from build123d import *

# Parameters (mm, degrees)
BOSS_EXTRUDE1_DEPTH = 40
FILLET1_R           = 20
SKETCH4_R           = 7.5
CUT_EXTRUDE1_DEPTH  = 40
CHAMFER1_SIZE       = 1


with BuildPart() as part:
    # Sketch3 → Boss-Extrude1 (new body)
    with BuildSketch(Plane.XY):
        with BuildLine():
            Line((-38.729833462, -5), (-100, -5))
            Line((-100, -5), (-100, 5))
            Line((-100, 5), (-38.729833462, 5))
            ThreePointArc((-38.729833462, 5), (-32.606109105, 7.09430585), (-29.047375097, 12.5))
            ThreePointArc((-29.047375097, 12.5), (0, 35), (29.047375097, 12.5))
            ThreePointArc((29.047375097, 12.5), (32.606109105, 7.09430585), (38.729833462, 5))
            Line((38.729833462, 5), (100, 5))
            Line((100, 5), (100, -5))
            Line((100, -5), (38.729833462, -5))
            ThreePointArc((38.729833462, -5), (32.606109105, -2.90569415), (29.047375097, 2.5))
            ThreePointArc((29.047375097, 2.5), (0, 25), (-29.047375097, 2.5))
            ThreePointArc((-29.047375097, 2.5), (-32.606109105, -2.90569415), (-38.729833462, -5))
        make_face()
    extrude(amount=BOSS_EXTRUDE1_DEPTH)

    # Fillet1
    fillet1_edges = [part.edges().sort_by_distance(p)[0] for p in [
        (100, 0, 0),
        (100, 0, 40),
        (-100, 0, 0),
        (-100, 0, 40),
    ]]
    fillet(fillet1_edges, radius=FILLET1_R - 0.0001)  # a hair under: the kernel refuses the full size

    # Sketch4 → Cut-Extrude1 (cut)
    with BuildSketch(Plane(origin=(0, 5, 0), x_dir=(1, 0, 0), z_dir=(0, 1, 0))):
        with Locations(Location((80, -20, 0), (0, 0, 180))):
            Circle(SKETCH4_R)
        with Locations(Location((-80, -20, 0), (0, 0, 180))):
            Circle(SKETCH4_R)
    extrude(amount=-CUT_EXTRUDE1_DEPTH, mode=Mode.SUBTRACT)

    # Chamfer1
    chamfer1_edges = [part.edges().sort_by_distance(p)[0] for p in [
        (87.5, 5, 20),
        (-72.5, 5, 20),
    ]]
    chamfer(chamfer1_edges, length=CHAMFER1_SIZE)


solid = part.part
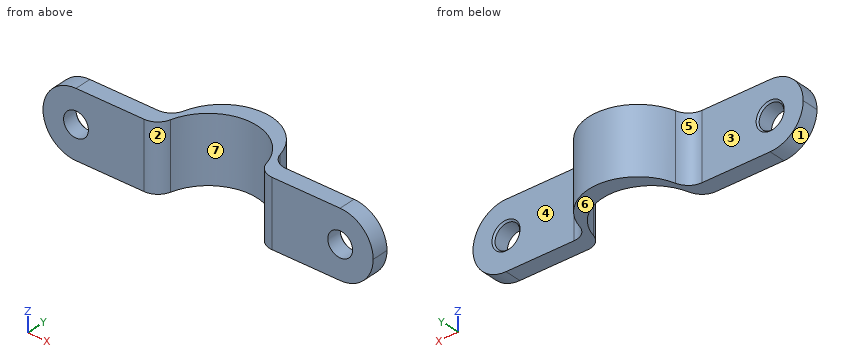
For this review, take the finished solid that the model builds, in its own axes (mm). Face numbers are marked on the shaded views. A direction names the side the tool comes from. Give positions to 0.01 mm unless a question says otherwise; leave off trailing zeros. Write each loop counter-clockwise with the first axis right and the second up, starting at its lowest first coordinate (ties: lowest second). Pieces come first, ordered by that corner, then holes. Notation, with made-up numbers: (-33, -12.75) -> (-12, -12.75) arc R15 cw to (-12, 5.25) -> close; hole circle Ø10 at (52, 71). An arc over 180 degrees is marked (long way). Use CSV: the item, a comma, the result in double quotes.
Q1. Take a section at B-B, the plane y = -1.5. State how many separate pieces and enclosed holes the cut face has, then the cut area to 3 significant figures.
Conclusion:
separate pieces,"2"
enclosed holes,"2"
area,"4,810 mm2"
Q2. Mouldability with a two-part tool opening along X and no side actions: class the marked faces 5, 6 and 7 as pulls with the +X half, pulls with the -X half, needs draft (parallel to the pull), parting line crosses it, or undercut.
Conclusion:
face 5,"pulls with the -X half"
face 6,"needs draft"
face 7,"undercut"
Q3. For P1, Ø10, axis at x = 33.5, y = 11.5, coming from the +Z side; P2, Ø4, axis at y = 3.5, z = 7, coming from the -X side; P3, Ø3, axis at y = 9.5, z = 29, coming from the -X side; P4, Ø6, axis at y = 22, z = 8.5, coming from the -X side, all flat-tipped, find the tip position at first contact; note any pin that passes through.
Conclusion:
P1,"z = 40"
P2,"x = -96.7"
P3,"x = -31.59"
P4,"x = -26.53"
Q4. Take a section at A-A, the plane y = 18.5. Write out the cut boundary in (x, z), then the cut area to 3 significant figures.
Conclusion:
outline,"(-26.79, 0) -> (-18.65, 0) -> (-18.65, 40) -> (-26.79, 40) -> close; (18.65, 0) -> (26.79, 0) -> (26.79, 40) -> (18.65, 40) -> close"
area,"651 mm2"
Q5. Take a section at C-C, the plane y = 9. Write out the cut boundary in (x, z).
Conclusion:
outline,"(-30.73, 0) -> (-26.53, 0) -> (-26.53, 40) -> (-30.73, 40) -> close; (26.53, 0) -> (30.73, 0) -> (30.73, 40) -> (26.53, 40) -> close"
Q6. Take a section at D-D, the plane x = 18.5. Write out the cut boundary in (y, z).
Conclusion:
outline,"(18.62, 0) -> (28.62, 0) -> (28.62, 40) -> (18.62, 40) -> close"
Q7. To check wall thickness, follow probe 1 along Z at (x, y) = (-80, 2.5); probe 2 along Y at (x, z) = (-69.5, 13.5); probe 3 along X at (y, z) = (4, 29). State the ranges of each line that lie inside material, in increasing order. Write a range as [from, to].
Conclusion:
probe 1,"[0, 12.5], [27.5, 40]"
probe 2,"[-5, 5]"
probe 3,"[-97.86, -28.62], [28.62, 97.86]"
Q8. Tool access review of the marked faces 1, 2, 3 and 4: name each direction out of +Z, -Z, +X, -X, +Y, -Y from which nothing blocks a thin tool from reaching the whole face with its end or side.
Conclusion:
face 1,"-Z, -X, +Y, -Y"
face 2,"+Z, -Z, -Y"
face 3,"+Z, -Z, -X, +Y"
face 4,"+Z, -Z, +X, +Y"
